Input: part model. Units: mm. Frame: model coordinates. Face numbers are marked on the shaded views. A direction names the side the tool comes from. Coordinates: 2 decimals unless noted, no trailing zeros. Loops run counter-clockwise (first coordinate to the right, second up) from the corner with the lowest first, then second, coordinate; pieces in that order, holes last.
Item 1: Contact query for flat-ended pins moving along their axis: P1, Ø10, axis at x = 5.5, z = 27.5, coming from the +Y side; P2, Ø3.5, axis at x = 12.5, y = -21.5, coming from the +Z side; P3, Ø8, axis at x = 25.5, z = 13, coming from the +Y side; P4, Ø3, axis at y = -27, z = 34.5, coming from the -X side. Output: stop coordinate, or through.
Item 2: Ray query, line 1 along Y through (x, z) = (7, 0); line 2 along Z through (x, y) = (11.5, 9.5); line 3 along Z through (x, y) = (27, 14.5). Return the intervals inside material, ascending.
Item 3: Reachability of the marked faces 1, 2 and 3 from +Z, -Z, +X, -X, +Y, -Y: full face, straight path, thin tool, end or side. Return the list, or none.
Item 4: Section B-B on z = 0. Return loops of the section in (x, y).
Item 5: Section A-A on x = 3.5. Return loops of the section in (y, z).
Item 6: Section C-C on y = 0. Return loops of the section in (x, z), and give its area (3 significant figures).
Item 7: Pull-direction query (Z, two-part tool) for the marked faces 4 and 5; classes: released by +Z, released by -Z, zero draft, split by the parting line, or undercut.
Item 8: Section D-D on x = 17.5. Return loops of the section in (y, z).
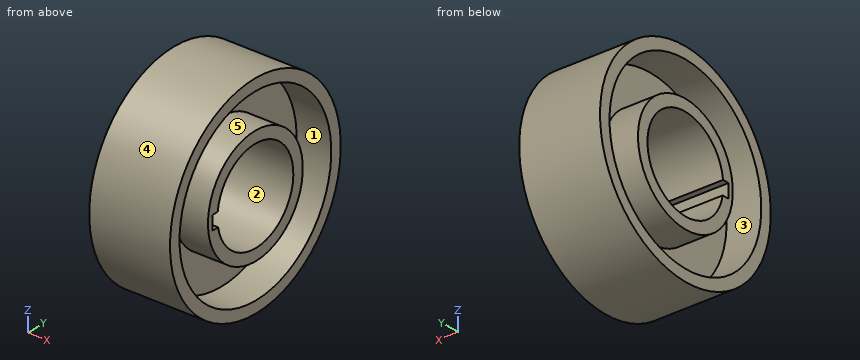
```python
from build123d import *

# Parameters (mm, degrees)
CUT_EXTRUDE1_START = -35
CUT_EXTRUDE1_DEPTH = 35
CUT_EXTRUDE2_DEPTH = 35


with BuildPart() as part:
    # Sketch2 → Revolve3 (revolve)
    with BuildSketch(Plane(origin=(0, 0, 0), x_dir=(1, 0, 0), z_dir=(0, 1, 0)), mode=Mode.PRIVATE) as revolve3_sk:
        Polygon((35, 20), (0, 20), (0, 25), (15, 25), (15, 40), (0, 40), (0, 45), (35, 45), (35, 40), (20, 40), (20, 25), (35, 25), align=None)
    revolve(revolve3_sk.sketch.rotate(Axis((0, 0, 0), (1, 0, 0)), 180), axis=Axis((0, 0, 0), (1, 0, 0)))

    # Sketch5 → Cut-Extrude1 (cut)
    with BuildSketch(Plane(origin=(35, 0, 0), x_dir=(0, 0, -1), z_dir=(1, 0, 0)).offset(CUT_EXTRUDE1_START)):
        with BuildLine():
            Line((-2.36724254, -19.85940993), (-2.36724254, -22.690863933))
            Line((-2.36724254, -22.690863933), (3.63275746, -22.690863933))
            Line((3.63275746, -22.690863933), (3.63275746, -19.85940993))
            Line((3.63275746, -19.85940993), (2.36724254, -19.85940993))
            ThreePointArc((2.36724254, -19.85940993), (0, -20), (-2.36724254, -19.85940993))
        make_face()
    extrude(amount=CUT_EXTRUDE1_DEPTH, mode=Mode.SUBTRACT)

    # Sketch6 → Cut-Extrude2 (cut)
    with BuildSketch(Plane(origin=(35, 0, 0), x_dir=(0, 0, -1), z_dir=(1, 0, 0))):
        Polygon((3.63275746, -19.85940993), (3.63275746, -19.592754897), (2.36724254, -19.85940993), align=None)
    extrude(amount=-CUT_EXTRUDE2_DEPTH, mode=Mode.SUBTRACT)


solid = part.part
```
Results found:
1. P1: stops at y = 38.97
1. P2: stops at z = 40.43
1. P3: stops at y = 44.09
1. P4: stops at x = 0
2. line 1: y = -45 to -40, -25 to -22.69, 20 to 25, 40 to 45
2. line 2: z = -43.99 to -38.86, -23.12 to -17.6, 17.6 to 23.12, 38.86 to 43.99
2. line 3: z = -42.6 to -37.28, -20.37 to -13.77, 13.77 to 20.37, 37.28 to 42.6
3. face 1: +X
3. face 2: +X, -X
3. face 3: -X
4. outline: (0, -45) - (35, -45) - (35, -40) - (20, -40) - (20, -25) - (35, -25) - (35, -22.69) - (0, -22.69) - (0, -25) - (15, -25) - (15, -40) - (0, -40) - close; (0, 20) - (35, 20) - (35, 25) - (20, 25) - (20, 40) - (35, 40) - (35, 45) - (0, 45) - (0, 40) - (15, 40) - (15, 25) - (0, 25) - close
5. outline: circle Ø90 at (0, 0); circle Ø50 at (0, 0); hole circle Ø80 at (0, 0); hole (-22.69, -3.63) - (-19.67, -3.63) arc R20 ccw (long way) to (-19.86, 2.37) - (-22.69, 2.37) - close
6. outline: (0, -45) - (35, -45) - (35, -40) - (20, -40) - (20, -25) - (35, -25) - (35, -20) - (0, -20) - (0, -25) - (15, -25) - (15, -40) - (0, -40) - close; (0, 20) - (35, 20) - (35, 25) - (20, 25) - (20, 40) - (35, 40) - (35, 45) - (0, 45) - (0, 40) - (15, 40) - (15, 25) - (0, 25) - close
6. area: 850 mm2
7. face 4: split by the parting line
7. face 5: undercut
8. outline: circle Ø90 at (0, 0); hole (-22.69, -3.63) - (-19.67, -3.63) arc R20 ccw (long way) to (-19.86, 2.37) - (-22.69, 2.37) - close
